Drawing for the job (mm, zero at the part's lowest x, y, z). A direction names the side the tool comes from. Coordinates: 2 decimals unless noted, no trailing zeros. Order: outer loops, then holes, each group sorted by start corner. A loop starts at its lowest first (then second) coordinate and runs counter-clockwise, first axis right, second up.
1) Cut at C-C (y = 16). List the corners of the cut face in (x, z).
2) Tool access for the marked faces 4 and 5: list every direction of +Z, -Z, +X, -X, +Y, -Y with a clear straight run to the whole face (end or side of a thin tool).
3) Pin check, flat tips, straight feed: pin 1 Ø5.5 at (x, y) = (15.5, 16) entering from -Z; pin 2 Ø4 at (x, y) = (15, 16) entering from +Z; pin 3 Ø6 at (x, z) = (6, 3.5) entering from -Y; pin 4 Ø5 at (x, z) = (12, 10.5) entering from -Y. Stop position of each tip, or through.
4) Cut at A-A (x = 15). Give the number of separate pieces and of enclosed holes in the cut face, and give its area (3 significant figures).
5) Mould opens along Z. For the marked faces 1, 2 and 3 say: +Z half, -Z half, draft (parallel to the pull), parting line (faces both ways), or undercut.
6) Cut at D-D (z = 6.75). List the corners of the cut face in (x, y).
7) Cut at B-B (y = 31). List the corners of the cut face in (x, z).
8) Wall check: L1, parallel to X at y = 16, z = 3.3; L2, parallel to X at y = 16, z = 0.5; L3, parallel to Z at x = 3, y = 31. Give the ranges that are in metal, low to high.
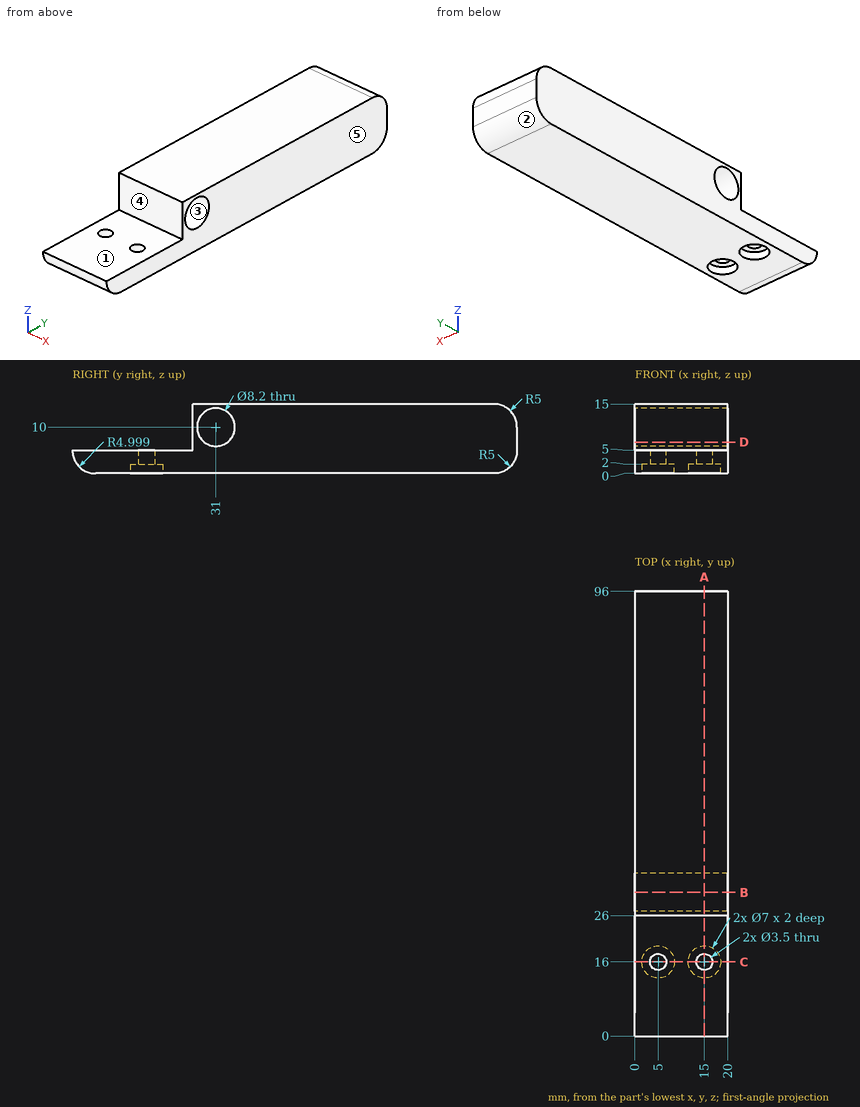
Geometry check:
1. outline: (0, 0) - (1.5, 0) - (1.5, 2) - (3.25, 2) - (3.25, 5) - (0, 5) - close; (6.75, 2) - (8.5, 2) - (8.5, 0) - (11.5, 0) - (11.5, 2) - (13.25, 2) - (13.25, 5) - (6.75, 5) - close; (16.75, 2) - (18.5, 2) - (18.5, 0) - (20, 0) - (20, 5) - (16.75, 5) - close
2. face 4: +Z, +X, -X, -Y
2. face 5: +Z, -Z, +X, +Y, -Y
3. pin 1: stops at z = 2
3. pin 2: stops at z = 5
3. pin 3: stops at y = 0
3. pin 4: stops at y = 26
4. separate pieces: 2
4. enclosed holes: 1
4. area: 1,090 mm2
5. face 1: +Z half
5. face 2: -Z half
5. face 3: undercut
6. outline: (0, 26) - (20, 26) - (20, 28.5) - (0, 28.5) - close; (0, 33.5) - (20, 33.5) - (20, 96) - (0, 96) - close
7. outline: (0, 0) - (20, 0) - (20, 5.9) - (0, 5.9) - close; (0, 14.1) - (20, 14.1) - (20, 15) - (0, 15) - close
8. L1: x = 0 to 3.25, 6.75 to 13.25, 16.75 to 20
8. L2: x = 0 to 1.5, 8.5 to 11.5, 18.5 to 20
8. L3: z = 0 to 5.9, 14.1 to 15
